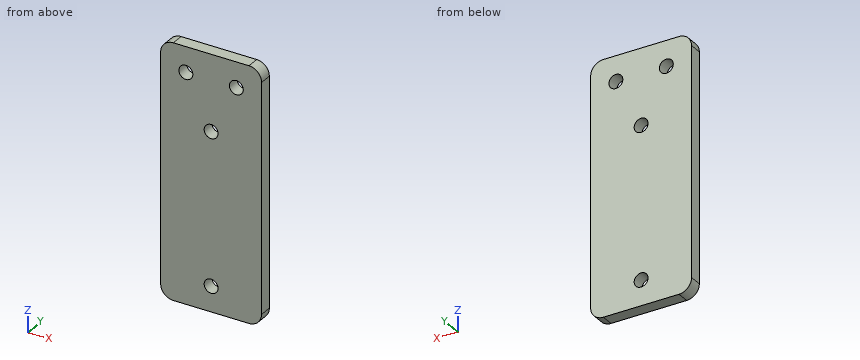
```python
from build123d import *

# Parameters (mm, degrees)
F0_W     = 40
F0_H     = 100
F1_DEPTH = 5
F2_R     = 5
F3_R     = 2.75
F4_DEPTH = 5.001


with BuildPart() as f1:
    # F0 (on Front) → F1 (new body)
    with BuildSketch(Plane.XZ):
        with Locations((20, 50)):
            Rectangle(F0_W, F0_H)
    extrude(amount=F1_DEPTH)

    # F2
    f2_edges = [f1.edges().sort_by_distance(p)[0] for p in [
        (0, -2.5, 100),
        (40, -2.5, 100),
        (40, -2.5, 0),
        (0, -2.5, 0),
    ]]
    fillet(f2_edges, radius=F2_R)


with BuildPart() as f4:
    # F3 (on Front) → F4 (new body, through all)
    with BuildSketch(Plane.XZ):
        with Locations((20, 10)):
            Circle(F3_R)
    extrude(amount=F4_DEPTH)


with BuildPart() as f1_1:
    add(f1.part)

    # F5: cut F4
    add(f4.part, mode=Mode.SUBTRACT)


with BuildPart() as f6_1:
    # F6: copy of F4
    add(f4.part.moved(Location((0, 0, 60))))


with BuildPart() as f7_1:
    # F7: copy of F6_1
    add(f6_1.part.moved(Location((10, 0, 20))))


with BuildPart() as f8_1:
    # F8: copy of F6_1
    add(f6_1.part.moved(Location((-10, 0, 20))))


with BuildPart() as f1_2:
    add(f1_1.part)

    # F9: cut F8_1, F7_1, F6_1, F4
    add(f8_1.part, mode=Mode.SUBTRACT)
    add(f7_1.part, mode=Mode.SUBTRACT)
    add(f6_1.part, mode=Mode.SUBTRACT)
    add(f4.part, mode=Mode.SUBTRACT)


solid = f1_2.part
```
Can you work these out from the model? Positions are in its coordinate system, mm. Coordinates: 2 decimals unless noted, no trailing zeros. Write each loop counter-clockwise with the first axis right and the second up, starting at its lowest first coordinate (ties: lowest second). Pieces come first, ordered by that corner, then holes. Notation, with made-up numbers: (-7, -31) - (9, -31) arc R15 cw to (9, -24) - close; hole circle Ø9 at (71, 54.5). An arc over 180 degrees is marked (long way). Return JSON: item names as keys, results as strings.
Q1. Please list where these lines run through material, in increasing order: L1, parallel to X at y = -2.8, z = 90; L2, parallel to Z at x = 20, y = -3.15; L3, parallel to Z at x = 21.5, y = -3.9. Write a range as from..to.
Computed values:
{"L1": "x = 0..7.25, 12.75..27.25, 32.75..40", "L2": "z = 0..7.25, 12.75..67.25, 72.75..100", "L3": "z = 0..7.7, 12.3..67.7, 72.3..100"}
Q2. If we section it at C-C (x = 20): Please give me the cut outline in (y, z), then the cut area to 3 significant figures.
Computed values:
{"outline": "(-5, 0) - (0, 0) - (0, 7.25) - (-5, 7.25) - close; (-5, 12.75) - (0, 12.75) - (0, 67.25) - (-5, 67.25) - close; (-5, 72.75) - (0, 72.75) - (0, 100) - (-5, 100) - close", "area": "445 mm2"}
Q3. If we section it at D-D (y = -0.85): Please give me the cut outline in (x, z), then the cut area to 3 significant figures.
Computed values:
{"outline": "(0, 5) arc R5 ccw to (5, 0) - (35, 0) arc R5 ccw to (40, 5) - (40, 95) arc R5 ccw to (35, 100) - (5, 100) arc R5 ccw to (0, 95) - close; hole circle Ø5.5 at (10, 90); hole circle Ø5.5 at (20, 10); hole circle Ø5.5 at (20, 70); hole circle Ø5.5 at (30, 90)", "area": "3,880 mm2"}
Q4. If we section it at A-A (x = 10): Please give me the cut outline in (y, z).
Computed values:
{"outline": "(-5, 0) - (0, 0) - (0, 87.25) - (-5, 87.25) - close; (-5, 92.75) - (0, 92.75) - (0, 100) - (-5, 100) - close"}
Q5. If we section it at B-B (z = 10): Please give me the cut outline in (x, y).
Computed values:
{"outline": "(0, -5) - (17.25, -5) - (17.25, 0) - (0, 0) - close; (22.75, -5) - (40, -5) - (40, 0) - (22.75, 0) - close"}
